Source: CAD feature listing. Evaluate the final solid. Frame: model axes, mm. Face numbers are marked on the shaded views. A direction names the side the tool comes from. Give positions to 0.01 mm unless a question says otherwise; leave off trailing zeros. Loops run counter-clockwise (first coordinate to the right, second up) from the corner with the lowest first, then second, coordinate; pieces in that order, holes last. Notation, with made-up numbers: M 15,8 L 65,8 A8 ccw 65,21 Z; hole C 33,77.5 d11. An arc over 180 degrees is marked long. Answer in a Markdown table with one row per item.
```python
from build123d import *

# Parameters (mm, degrees)
SKIZZE1_W                         = 48
SKIZZE1_H                         = 48
AUFSATZ_LINEAR_AUSTRAGEN1_DEPTH   = 2
LINEAR_AUSTRAGEN_D_NN1_DEPTH      = 26
LINEAR_AUSTRAGEN_D_NN1_DEPTH_BACK = 2
SKIZZE2_W                         = 52
SKIZZE2_H                         = 52
SKIZZE2_W_2                       = 48
SKIZZE2_H_2                       = 48
SCHNITT_LINEAR_AUSTRAGEN1_REACH   = 66.529
SKIZZE4_W                         = 10
SKIZZE4_H                         = 3.5
SCHNITT_LINEAR_AUSTRAGEN2_REACH   = 66.529
SKIZZE5_W                         = 2.4
SKIZZE5_H                         = 2.4
SKIZZE6_W                         = 3
SKIZZE6_H                         = 4.8
AUFSATZ_LINEAR_AUSTRAGEN2_DEPTH   = 19.1
SKIZZE7_W                         = 3.6
SKIZZE7_H                         = 2.4
AUFSATZ_LINEAR_AUSTRAGEN3_DEPTH   = 20.6
SKIZZE8_W                         = 0.6
SKIZZE8_H                         = 2.4
AUFSATZ_LINEAR_AUSTRAGEN4_DEPTH   = 2
SKIZZE9_W                         = 37
SKIZZE9_H                         = 2.6
AUFSATZ_LINEAR_AUSTRAGEN5_DEPTH   = 20.6
AUFSATZ_LINEAR_AUSTRAGEN6_DEPTH   = 26
SKIZZE11_W                        = 37
SKIZZE11_H                        = 2.8
AUFSATZ_LINEAR_AUSTRAGEN7_DEPTH   = 24


with BuildPart() as part:
    # Skizze1 → Aufsatz-Linear austragen1 (new body)
    with BuildSketch(Plane(origin=(0, 0, 0), x_dir=(1, 0, 0), z_dir=(0, 1, 0))):
        Rectangle(SKIZZE1_W, SKIZZE1_H)
    extrude(amount=AUFSATZ_LINEAR_AUSTRAGEN1_DEPTH)

    # Skizze2 → Linear-Austragen-Dünn1 (add, two sides: drawn at the far end of the back side and taken through both)
    with BuildSketch(Plane(origin=(0, 2, 0), x_dir=(1, 0, 0), z_dir=(0, 1, 0)).offset(-LINEAR_AUSTRAGEN_D_NN1_DEPTH_BACK)):
        Rectangle(SKIZZE2_W, SKIZZE2_H)
        Rectangle(SKIZZE2_W_2, SKIZZE2_H_2, mode=Mode.SUBTRACT)
    extrude(amount=LINEAR_AUSTRAGEN_D_NN1_DEPTH + LINEAR_AUSTRAGEN_D_NN1_DEPTH_BACK)

    # Skizze4 → Schnitt-Linear austragen1 (cut, up to next)
    with BuildSketch(Plane(origin=(0, 0, -26), x_dir=(-1, 0, 0), z_dir=(0, 0, -1)), mode=Mode.PRIVATE) as schnitt_linear_austragen1_sk1:
        with Locations((-12.2, 21.95)):
            Rectangle(SKIZZE4_W, SKIZZE4_H)
    schnitt_linear_austragen1_tool1 = extrude(schnitt_linear_austragen1_sk1.sketch, amount=-SCHNITT_LINEAR_AUSTRAGEN1_REACH, mode=Mode.PRIVATE) & part.part
    add(schnitt_linear_austragen1_tool1.solids().sort_by_distance((12.2, 21.95, -26))[0], mode=Mode.SUBTRACT)

    # Skizze5 → Schnitt-Linear austragen2 (cut, up to next)
    with BuildSketch(Plane(origin=(26, 0, 0), x_dir=(0, 0, -1), z_dir=(1, 0, 0)), mode=Mode.PRIVATE) as schnitt_linear_austragen2_sk1:
        with Locations((21.4, 22.4)):
            Rectangle(SKIZZE5_W, SKIZZE5_H)
    schnitt_linear_austragen2_tool1 = extrude(schnitt_linear_austragen2_sk1.sketch, amount=-SCHNITT_LINEAR_AUSTRAGEN2_REACH, mode=Mode.PRIVATE) & part.part
    add(schnitt_linear_austragen2_tool1.solids().sort_by_distance((26, 22.4, -21.4))[0], mode=Mode.SUBTRACT)

    # Skizze6 → Aufsatz-Linear austragen2 (add)
    with BuildSketch(Plane(origin=(0, 2, 0), x_dir=(1, 0, 0), z_dir=(0, 1, 0))):
        with Locations((20.5, 19)):
            Rectangle(SKIZZE6_W, SKIZZE6_H)
    extrude(amount=AUFSATZ_LINEAR_AUSTRAGEN2_DEPTH)

    # Skizze7 → Aufsatz-Linear austragen3 (add)
    with BuildSketch(Plane(origin=(0, 2, 0), x_dir=(1, 0, 0), z_dir=(0, 1, 0))):
        with Locations((-0.6, 22.8)):
            Rectangle(SKIZZE7_W, SKIZZE7_H)
    extrude(amount=AUFSATZ_LINEAR_AUSTRAGEN3_DEPTH)

    # Skizze8 → Aufsatz-Linear austragen4 (add)
    with BuildSketch(Plane(origin=(0, 22.6, 0), x_dir=(1, 0, 0), z_dir=(0, 1, 0))):
        with Locations((-2.1, 22.8)):
            Rectangle(SKIZZE8_W, SKIZZE8_H)
    extrude(amount=AUFSATZ_LINEAR_AUSTRAGEN4_DEPTH)

    # Skizze9 → Aufsatz-Linear austragen5 (add)
    with BuildSketch(Plane(origin=(0, 2, 0), x_dir=(1, 0, 0), z_dir=(0, 1, 0))):
        with Locations((5.5, -9.2)):
            Rectangle(SKIZZE9_W, SKIZZE9_H)
    extrude(amount=AUFSATZ_LINEAR_AUSTRAGEN5_DEPTH)

    # Skizze10 → Aufsatz-Linear austragen6 (add)
    with BuildSketch(Plane(origin=(0, 2, 0), x_dir=(1, 0, 0), z_dir=(0, 1, 0))):
        Polygon((-24, 21.6), (-21.6, 21.6), (-21.6, 24), (-20, 24), (-20, 20), (-24, 20), align=None)
        Polygon((-24, -21.6), (-21.6, -21.6), (-21.6, -24), (-20, -24), (-20, -20), (-24, -20), align=None)
    extrude(amount=AUFSATZ_LINEAR_AUSTRAGEN6_DEPTH)

    # Skizze11 → Aufsatz-Linear austragen7 (add)
    with BuildSketch(Plane(origin=(0, 2, 0), x_dir=(1, 0, 0), z_dir=(0, 1, 0))):
        with Locations((5.5, -11.9)):
            Rectangle(SKIZZE11_W, SKIZZE11_H)
    extrude(amount=AUFSATZ_LINEAR_AUSTRAGEN7_DEPTH)


solid = part.part
```
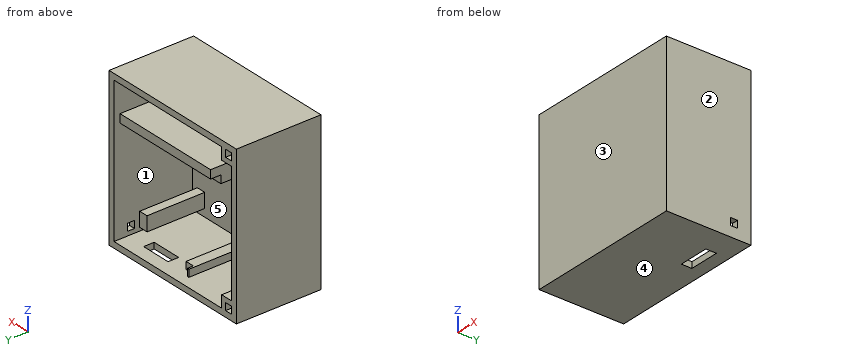
1) Material intervals for L1, parallel to X at y = 7, z = -18.5; L2, parallel to Z at x = 13.5, y = 10.25; L3, parallel to Z at x = 0, y = 20.5, sorted ascending.
Reply:
| item | result |
|---|---|
| L1 | x = -26 to -24, 19 to 22, 24 to 26 |
| L2 | z = -26 to -24, 7.9 to 13.3, 24 to 26 |
| L3 | z = -26 to -21.6, 7.9 to 13.3, 24 to 26 |
2) Section C-C, the plane x = 20.5. Return loops of the section in (y, z), then the cut area to 3 significant figures.
Reply:
| item | result |
|---|---|
| outline | M 0,-26 L 28,-26 L 28,-24 L 2,-24 L 2,-21.4 L 21.1,-21.4 L 21.1,-16.6 L 2,-16.6 L 2,7.9 L 22.6,7.9 L 22.6,10.5 L 26,10.5 L 26,13.3 L 2,13.3 L 2,24 L 28,24 L 28,26 L 0,26 Z |
| area | 420 mm² |
3) Section A-A, the plane y = 11. Count the separate pieces of the cut face and the enclosed holes in it, then the cut area to 3 significant figures.
Reply:
| item | result |
|---|---|
| separate pieces | 2 |
| enclosed holes | 3 |
| area | 643 mm² |
4) Pull-direction query (Z, two-part tool) for the marked faces 3, 4 and 5; classes: released by +Z, released by -Z, zero draft, split by the parting line, or undercut.
Reply:
| item | result |
|---|---|
| face 3 | zero draft |
| face 4 | released by -Z |
| face 5 | undercut |
5) Section B-B, the plane x = 13. Return loops of the section in (y, z).
Reply:
| item | result |
|---|---|
| outline | M 0,-26 L 20.2,-26 L 20.2,-24 L 2,-24 L 2,7.9 L 22.6,7.9 L 22.6,10.5 L 26,10.5 L 26,13.3 L 2,13.3 L 2,24 L 28,24 L 28,26 L 0,26 Z; M 23.7,-26 L 28,-26 L 28,-24 L 23.7,-24 Z |
6) Section D-D, the plane z = 4. Return loops of the section in (x, y), then the cut area to 3 significant figures.
Reply:
| item | result |
|---|---|
| outline | M -26,0 L 26,0 L 26,28 L 24,28 L 24,2 L -24,2 L -24,28 L -26,28 Z |
| area | 208 mm² |
7) Pin query (flat end, axial travel): pin 1 Ø6 at (x, z) = (17, -11) entering from -Y; pin 2 Ø1.5 at (x, z) = (14.5, 18.5) entering from +Y. Return the tip coordinate at first contact, or that it passes through.
Reply:
| item | result |
|---|---|
| pin 1 | stops at y = 0 |
| pin 2 | stops at y = 2 |
8) Set-up query: the marked faces 1 and 2. Return all of +Z, -Z, +X, -X, +Y, -Y with unobstructed straight access to the full face (end or side cutting, diameter ignored); none if empty.
Reply:
| item | result |
|---|---|
| face 1 | +Y |
| face 2 | +Z, -Z, +X, +Y, -Y |
